CAD build for the part. Positions are in the model's coordinates, mm. A direction names the side the tool comes from. Give positions to 0.01 mm unless a question says otherwise; leave off trailing zeros. Order: outer loops, then holes, each group sorted by start corner. A loop starts at its lowest first (then second) coordinate and runs counter-clockwise, first axis right, second up.
Item 1: Two-plate mould, pull along Y, no slides. Class faces 4 (the flat face through (9, 16, 5)), 5 (the cylindrical face through (9.62, 2.85, 3.01)), 6 (the cylindrical face through (9.619, 24.735, 0.782)): released by +Y, released by -Y, zero draft, split by the parting line, or undercut.
Item 2: Which spindle directions (+Z, -Z, +X, -X, +Y, -Y) get a long thin tool onto all of the face, cutting with end or side? Do faces 1 (the cylindrical face through (18.248, 33.32, 11.885)), 2 (the cylindrical face through (9.619, 22.797, 5.391)), 3 (the cylindrical face through (0.3, 27.59, 9.26)). Say none if no direction does.
Item 3: Band-saw the part on B-B on z = 25. Give the cut face in (x, y).
Item 4: Band-saw the part on A-A on x = 6. Give the cut face in (y, z).
Item 5: Flat gauge pins, fed straight in: P1, Ø3, axis at x = 7.5, y = 59.5, coming from the +Z side; P2, Ø8, axis at x = 12.5, z = 29.5, coming from the +Y side; P3, Ø5.5, axis at x = 6.5, y = 17, coming from the +Z side. Where does each tip first touch, or does it go through?
Item 6: Wall check: L1, parallel to Y at x = 15.25, z = 16; L2, parallel to Y at x = 3.5, z = 13; L3, parallel to Z at x = 11.5, y = 16. Give the ranges that are in metal, low to high.
```python
from build123d import *

# Parameters (mm, degrees)
F1_DEPTH        = 19
F2_R            = 10
F3_R            = 10
F4_R            = 5
F5_R            = 5
F6_R            = 10
F7_R            = 5
F8_R            = 2.5
F9_R            = 1
F11_D           = 4
F11_CSINK_D     = 6
F11_CSINK_ANGLE = 45
F12_D           = 4
F12_CSINK_D     = 6
F12_CSINK_ANGLE = 45


with BuildPart() as f1:
    # F0 (on Right) → F1 (new body)
    with BuildSketch(Plane.YZ):
        Polygon((0, 60), (0, 0), (25, 0), (35.606602, 10.606602), (32.071068, 14.142136), (22.928932, 5), (5, 5), (5, 57.113249), (71.782032, 95.669873), (69.282032, 100), align=None)
    extrude(amount=F1_DEPTH)

    # F2
    f2_edges = [f1.edges().sort_by_distance(p)[0] for p in [
        (9.5, 0, 60),
    ]]
    fillet(f2_edges, radius=F2_R)

    # F3
    f3_edges = [f1.edges().sort_by_distance(p)[0] for p in [
        (9.5, 0, 0),
    ]]
    fillet(f3_edges, radius=F3_R)

    # F4
    f4_edges = [f1.edges().sort_by_distance(p)[0] for p in [
        (9.5, 5, 5),
    ]]
    fillet(f4_edges, radius=F4_R)

    # F5
    f5_edges = [f1.edges().sort_by_distance(p)[0] for p in [
        (9.5, 5, 57.113249),
    ]]
    fillet(f5_edges, radius=F5_R)

    # F6
    f6_edges = [f1.edges().sort_by_distance(p)[0] for p in [
        (9.5, 25, 0),
    ]]
    fillet(f6_edges, radius=F6_R)

    # F7
    f7_edges = [f1.edges().sort_by_distance(p)[0] for p in [
        (9.5, 22.928932, 5),
    ]]
    fillet(f7_edges, radius=F7_R)

    # F8
    f8_edges = [f1.edges().sort_by_distance(p)[0] for p in [
        (19, 33.838835, 12.374369),
        (0, 33.838835, 12.374369),
        (0, 70.532032, 97.834936),
        (19, 70.532032, 97.834936),
    ]]
    fillet(f8_edges, radius=F8_R)

    # F9
    f9_edges = [f1.edges().sort_by_distance(p)[0] for p in [
        (9.5, 35.606602, 10.606602),
        (9.5, 32.071068, 14.142136),
    ]]
    fillet(f9_edges, radius=F9_R)

    # F11 (through all)
    with Locations(Plane(origin=(0, 5, 0), x_dir=(-1, 0, 0), z_dir=(0, 1, 0))):
        with Locations((-14.348798, 48.270144)):
            CounterSinkHole(F11_D / 2, F11_CSINK_D / 2, counter_sink_angle=F11_CSINK_ANGLE)

    # F12 (through all)
    with Locations(Plane(origin=(0, 5, 0), x_dir=(-1, 0, 0), z_dir=(0, 1, 0))):
        with Locations((-6, 34.226497)):
            CounterSinkHole(F12_D / 2, F12_CSINK_D / 2, counter_sink_angle=F12_CSINK_ANGLE)


solid = f1.part
```
The answers:
1. face 4: undercut
1. face 5: released by -Y
1. face 6: released by +Y
2. face 1: +X, +Y
2. face 2: +X, -X
2. face 3: -X
3. outline: (0, 1) arc R1 ccw to (1, 0) - (18, 0) arc R1 ccw to (19, 1) - (19, 4) arc R1 ccw to (18, 5) - (1, 5) arc R1 ccw to (0, 4) - close
4. outline: (0, 10) arc R10 ccw to (10, 0) - (20.86, 0) arc R10 ccw to (27.93, 2.93) - (34.9, 9.9) arc R1 ccw to (34.9, 11.31) - (32.78, 13.44) arc R1 ccw to (31.36, 13.44) - (24.39, 6.46) arc R5 cw to (20.86, 5) - (10, 5) arc R5 cw to (5, 10) - (5, 31.23) - (2.59, 32.23) - (0, 32.23) - close; (0, 36.23) - (2.59, 36.23) - (5, 37.23) - (5, 54.23) arc R5 cw to (7.5, 58.56) - (70.92, 95.17) arc R1 ccw to (71.28, 96.54) - (69.78, 99.13) arc R1 ccw to (68.42, 99.5) - (5, 62.89) arc R10 ccw to (0, 54.23) - close
5. P1: stops at z = 95.22
5. P2: stops at y = 5
5. P3: stops at z = 71.4
6. L1: y = 0 to 5
6. L2: y = 0 to 5, 30.93 to 33.21
6. L3: z = 0 to 5, 63.46 to 69.24
